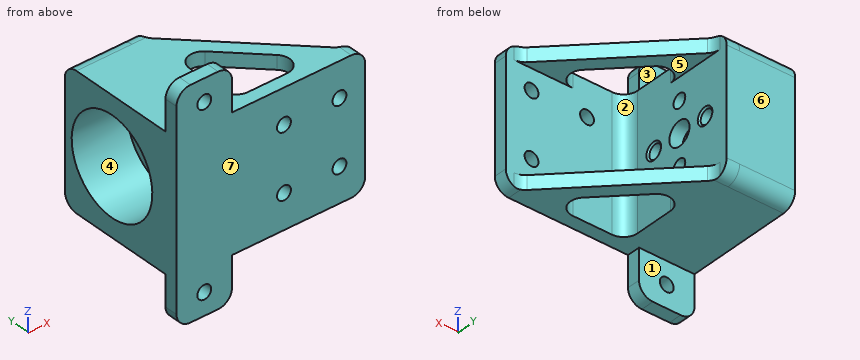
```python
from build123d import *

# Parameters (mm, degrees)
SKETCH1_W                      = 30.48
SKETCH1_H                      = 30.48
BOSS_EXTRUDE1_DEPTH            = 30.48
SKETCH2_W                      = 27.48
SKETCH2_H                      = 27.48
CUT_EXTRUDE1_DEPTH             = 46.72
F_10_CLEARANCE_HOLE1_D         = 5.5
F_4_CLEARANCE_HOLE1_D          = 3.2
CHAMFER1_SIZE                  = 0.399999962
CHAMFER1_SIZE2                 = 0.335639821
FILLET1_R                      = 3.175
BOSS_EXTRUDE2_DEPTH            = 3.175
SKETCH20_R                     = 11
BOSS_EXTRUDE3_DEPTH            = 12.7
SKETCH21_W                     = 12.7
SKETCH21_H                     = 50.8
BOSS_EXTRUDE4_DEPTH            = 3
FILLET2_R                      = 3.175
F_1_8_0_1250_DOWEL_HOLE1_D     = 3.175
F_1_8_0_1250_DOWEL_HOLE1_DEPTH = 6.35
F_1_8_0_1250_DOWEL_HOLE1_TIP   = 0.953866233
F_1_8_0_1250_DOWEL_HOLE2_D     = 3.175
F_1_8_0_1250_DOWEL_HOLE2_DEPTH = 6.35
F_1_8_0_1250_DOWEL_HOLE2_TIP   = 0.953866233


with BuildPart() as part:
    # Sketch1 → Boss-Extrude1 (new body)
    with BuildSketch(Plane.XZ):
        Rectangle(SKETCH1_W, SKETCH1_H)
    extrude(amount=-BOSS_EXTRUDE1_DEPTH)

    # Sketch2 → Cut-Extrude1 (cut, through all)
    with BuildSketch(Plane(origin=(0, 0, -15.24), x_dir=(-1, 0, 0), z_dir=(0, 0, -1))):
        with Locations((-1.5, 16.74)):
            Rectangle(SKETCH2_W, SKETCH2_H)
    extrude(amount=-CUT_EXTRUDE1_DEPTH, mode=Mode.SUBTRACT)

    # #10 Clearance Hole1 (through all)
    with Locations(Plane(origin=(-12.24, 0, 0), x_dir=(0, 0, -1), z_dir=(1, 0, 0))):
        with Locations((0, 17.605)):
            Hole(F_10_CLEARANCE_HOLE1_D / 2)

    # #4 Clearance Hole1 (through all)
    with Locations(Plane(origin=(-12.24, 0, 0), x_dir=(0, 0, -1), z_dir=(1, 0, 0))):
        with Locations((-7, 17.605), (7, 17.605), (0, 24.605), (0, 10.605)):
            Hole(F_4_CLEARANCE_HOLE1_D / 2)

    # Chamfer1
    chamfer1_edges = [part.edges().sort_by_distance(p)[0] for p in [
        (-12.24, 10.605, -1.6),
        (-12.24, 24.605, -1.6),
    ]]
    chamfer1_side = [part.faces().sort_by_distance(p)[0] for p in [
        (-12.24, 16.74, -14.829612281),
    ]]
    chamfer(chamfer1_edges, length=CHAMFER1_SIZE, length2=CHAMFER1_SIZE2, reference=chamfer1_side[0])

    # Fillet1
    fillet1_edges = [part.edges().sort_by_distance(p)[0] for p in [
        (-13.74, 30.48, 15.24),
        (15.24, 1.5, -15.24),
        (15.24, 1.5, 15.24),
        (-12.24, 3, 0),
        (-13.74, 30.48, -15.24),
    ]]
    fillet(fillet1_edges, radius=FILLET1_R)

    # Sketch11 → Boss-Extrude2 (add)
    with BuildSketch(Plane.XY.offset(15.24)):
        Polygon((-12.24, 27.305), (12.065, 3), (7.574871939, 3), (-12.24, 22.814871939), align=None)
    boss_extrude2 = extrude(amount=-BOSS_EXTRUDE2_DEPTH)

    # Mirror1: Boss-Extrude2 across plane
    add(boss_extrude2.mirror(Plane(origin=(0, 0, 0), x_dir=(1, 0, 0), z_dir=(0, 0, -1))))

    # Sketch20 → Boss-Extrude3 (add)
    with BuildSketch(Plane.ZY.offset(15.24)):
        with BuildLine():
            Line((15.24, 0), (15.24, 27.305))
            ThreePointArc((15.24, 27.305), (14.31006403, 29.55006403), (12.065, 30.48))
            Line((12.065, 30.48), (-12.065, 30.48))
            ThreePointArc((-12.065, 30.48), (-14.31006403, 29.55006403), (-15.24, 27.305))
            Line((-15.24, 27.305), (-15.24, 0))
            Line((-15.24, 0), (15.24, 0))
        make_face()
        with Locations((0, 17.605)):
            Circle(SKETCH20_R, mode=Mode.SUBTRACT)
    extrude(amount=BOSS_EXTRUDE3_DEPTH)

    # Sketch21 → Boss-Extrude4 (add)
    with BuildSketch(Plane.XZ):
        with Locations((-21.59, 0)):
            Rectangle(SKETCH21_W, SKETCH21_H)
    extrude(amount=-BOSS_EXTRUDE4_DEPTH)

    # Fillet2
    fillet2_edges = [part.edges().sort_by_distance(p)[0] for p in [
        (-12.24, 27.305, -13.6525),
        (-12.24, 22.814871939, -13.6525),
        (7.574871939, 3, -13.6525),
        (12.065, 3, -13.6525),
        (-15.24, 1.5, 25.4),
        (-27.94, 1.5, -25.4),
        (-27.94, 1.5, 25.4),
        (-15.24, 1.5, -25.4),
        (-12.24, 22.814871939, 13.6525),
        (-12.24, 27.305, 13.6525),
        (12.065, 3, 13.6525),
        (7.574871939, 3, 13.6525),
    ]]
    fillet(fillet2_edges, radius=FILLET2_R)

    # 1/8 (0.1250) Dowel Hole1
    with Locations(Plane(origin=(0, 3, 0), x_dir=(1, 0, 0), z_dir=(0, 1, 0))):
        with Locations((-3.35, 7.29577013), (9.35, 7.29577013), (9.35, -7.29577013), (-3.35, -7.29577013)):
            Hole(F_1_8_0_1250_DOWEL_HOLE1_D / 2, depth=F_1_8_0_1250_DOWEL_HOLE1_DEPTH)
            with Locations((0, 0, -(F_1_8_0_1250_DOWEL_HOLE1_DEPTH + F_1_8_0_1250_DOWEL_HOLE1_TIP / 2))):  # 118° drill point
                Cone(0, F_1_8_0_1250_DOWEL_HOLE1_D / 2, F_1_8_0_1250_DOWEL_HOLE1_TIP, mode=Mode.SUBTRACT)

    # 1/8 (0.1250) Dowel Hole2
    with Locations(Plane(origin=(0, 3, 0), x_dir=(1, 0, 0), z_dir=(0, 1, 0))):
        with Locations((-21.59, 20.32), (-21.59, -20.32)):
            Hole(F_1_8_0_1250_DOWEL_HOLE2_D / 2, depth=F_1_8_0_1250_DOWEL_HOLE2_DEPTH)
            with Locations((0, 0, -(F_1_8_0_1250_DOWEL_HOLE2_DEPTH + F_1_8_0_1250_DOWEL_HOLE2_TIP / 2))):  # 118° drill point
                Cone(0, F_1_8_0_1250_DOWEL_HOLE2_D / 2, F_1_8_0_1250_DOWEL_HOLE2_TIP, mode=Mode.SUBTRACT)


solid = part.part
```
Could you check a few things on this model? Use its own coordinates, in mm. Face numbers are marked on the shaded views. A direction names the side the tool comes from. Coordinates: 2 decimals unless noted, no trailing zeros. Write each loop counter-clockwise with the first axis right and the second up, starting at its lowest first coordinate (ties: lowest second). Pieces come first, ordered by that corner, then holes. Notation, with made-up numbers: (52.25, 67.25) -> (63.25, 67.25) arc R28 cw to (63.25, 91.25) -> close; hole circle Ø10 at (22, 39.25). An arc over 180 degrees is marked (long way). One line per question, with ' | ' between items. Start each with the question number.
1. If we section it at B-B (x = -21.59): Count the separate pieces of the cut face and the enclosed holes in it, and give its area (3 significant figures).
2. If we section it at A-A (z = -20.32): Please give me the cut outline in (x, y).
3. If we section it at D-D (x = -3.35): Please give me the cut outline in (y, z) (3 decimals).
4. If we section it at C-C (z = 0): Please give me the cut outline in (x, y) (3 decimals), and give its area (3 significant figures).
5. For the marked faces 1, 2 and 3, which set-ups out of +Z, -Z, +X, -X, +Y, -Y let a thin tool reach every point of the face, with its end or its side?
6. Will these pins go through, and if not, where does the flat tip stop? P1, Ø5, axis at x = -21.59, z = -20.32, coming from the +Y side; P2, Ø11, axis at x = -20.5, z = 19.5, coming from the +Y side; P3, Ø4, axis at y = 17.605, z = -7, coming from the +X side.
7. Thinking about a two-plate mould opening in Y: for the marked faces 4, 5, 6 and 7, which applies, pulls with the +Y half, pulls with the -Y half, needs draft (parallel to the pull), parting line crosses it, or undercut?
8. Please list where these lines run through material, in increasing order: line 1 along Z through (x, y) = (-21.59, 0.8); line 2 along Y through (x, z) = (-19, 0) (3 decimals); line 3 along X through (y, z) = (0.95, -20.32).
Return value:
1) separate pieces: 3 | enclosed holes: 1 | area: 586 mm²
2) outline: (-27.94, 0) -> (-23.18, 0) -> (-23.18, 3) -> (-27.94, 3) -> close; (-20, 0) -> (-15.24, 0) -> (-15.24, 3) -> (-20, 3) -> close
3) outline: (0, -15.24) -> (3, -15.24) -> (3, -8.883) -> (0, -8.883) -> close; (0, -5.708) -> (3, -5.708) -> (3, 5.708) -> (0, 5.708) -> close; (0, 8.883) -> (3, 8.883) -> (3, 15.24) -> (0, 15.24) -> close; (13.925, -15.24) -> (18.415, -15.24) -> (18.415, -12.065) -> (13.925, -12.065) -> close; (13.925, 12.065) -> (18.415, 12.065) -> (18.415, 15.24) -> (13.925, 15.24) -> close
4) outline: (-27.94, 0) -> (15.24, 0) -> (15.24, 3) -> (-9.065, 3) arc R3.175 cw to (-12.24, 6.175) -> (-12.24, 8.605) -> (-12.576, 9.005) -> (-15.24, 9.005) -> (-15.24, 6.605) -> (-27.94, 6.605) -> close; (-27.94, 28.605) -> (-15.24, 28.605) -> (-15.24, 26.205) -> (-12.576, 26.205) -> (-12.24, 26.605) -> (-12.24, 30.48) -> (-27.94, 30.48) -> close; (-15.24, 12.205) -> (-12.576, 12.205) -> (-12.24, 12.605) -> (-12.24, 14.855) -> (-15.24, 14.855) -> close; (-15.24, 20.355) -> (-12.24, 20.355) -> (-12.24, 22.605) -> (-12.576, 23.005) -> (-15.24, 23.005) -> close | area: 248 mm²
5) face 1: -Z, +X, -X, +Y | face 2: +Z, -Z | face 3: +Z, +X, -X, +Y
6) P1: stops at y = 3 | P2: stops at y = 29.82 | P3: stops at x = -12.24
7) face 4: undercut | face 5: needs draft | face 6: pulls with the +Y half | face 7: pulls with the -Y half
8) line 1: z = -25.4 to -21.91, -18.73 to 18.73, 21.91 to 25.4 | line 2: y = 0 to 6.605, 28.605 to 30.48 | line 3: x = -27.94 to -23.18, -20 to -15.24
